Verification items for the finished model (mm, model axes). A direction names the side the tool comes from. Round coordinates to 2 decimals unless told otherwise and drop trailing zeros. Loops run counter-clockwise (first coordinate to the right, second up) from the corner with the lowest first, then second, coordinate; pieces in that order, holes last. Notation, with made-up numbers: M 71.5,-19 L 113.5,-19 A27 ccw 113.5,9 Z; hole C 19,58 d3. An arc over 180 degrees is marked long. Write item = value, one per line. Start each with the question number.
from build123d import *

# Parameters (mm, degrees)
ESQUISSE1_W             = 30
ESQUISSE1_H             = 30
BOSS_EXTRU_1_DEPTH      = 30
ESQUISSE2_W             = 20
ESQUISSE2_H             = 20
ENL_V_MAT_EXTRU_1_DEPTH = 31
ESQUISSE3_W             = 20
ESQUISSE3_H             = 20
ENL_V_MAT_EXTRU_2_DEPTH = 31
ESQUISSE4_W             = 20
ESQUISSE4_H             = 20
ENL_V_MAT_EXTRU_3_DEPTH = 31


with BuildPart() as part:
    # Esquisse1 → Boss.-Extru.1 (new body)
    with BuildSketch(Plane.XY):
        with Locations((15, 15)):
            Rectangle(ESQUISSE1_W, ESQUISSE1_H)
    extrude(amount=BOSS_EXTRU_1_DEPTH)

    # Esquisse2 → Enlèv. mat.-Extru.1 (cut, through all)
    with BuildSketch(Plane(origin=(0, 30, 0), x_dir=(1, 0, 0), z_dir=(0, 1, 0))):
        with Locations((15, -15)):
            Rectangle(ESQUISSE2_W, ESQUISSE2_H)
    extrude(amount=-ENL_V_MAT_EXTRU_1_DEPTH, mode=Mode.SUBTRACT)

    # Esquisse3 → Enlèv. mat.-Extru.2 (cut, through all)
    with BuildSketch(Plane.XY.offset(30)):
        with Locations((15, 15)):
            Rectangle(ESQUISSE3_W, ESQUISSE3_H)
    extrude(amount=-ENL_V_MAT_EXTRU_2_DEPTH, mode=Mode.SUBTRACT)

    # Esquisse4 → Enlèv. mat.-Extru.3 (cut, through all)
    with BuildSketch(Plane(origin=(30, 0, 0), x_dir=(0, 0, -1), z_dir=(1, 0, 0))):
        with Locations((-15, 15)):
            Rectangle(ESQUISSE4_W, ESQUISSE4_H)
    extrude(amount=-ENL_V_MAT_EXTRU_3_DEPTH, mode=Mode.SUBTRACT)


solid = part.part
1. Tool access check on faces 1 (the flat face through (3, 15, 25)), 2 (the flat face through (25, 15, 3)), 3 (the flat face through (25, 3, 15)). Record the directions out of +Z, -Z, +X, -X, +Y, -Y that give a thin tool (end or side, any length) a straight path to the whole face; none if there is none.
2. Section check C-C, the plane x = 27.5. Enter the section's corners in (y, z), and give its area (3 significant figures).
3. Gauge pin test, flat end, axial feed: P1, Ø4, axis at x = 8, z = 16, coming from the -Y side. Record the tip position at first contact, or that the pin passes through.
4. Section check A-A, the plane z = 8.5. Enter the section's corners in (x, y).
5. Mould release check, pull along Z, two halves, no side actions. Record for faces 4 (the flat face through (4.8, 15.2, 30)), 5 (the flat face through (15, 5, 28)), 6 (the flat face through (5, 28, 15)), 7 (the flat face through (3, 5, 15)): pulls with the +Z half, pulls with the -Z half, needs draft (parallel to the pull), parting line crosses it, or undercut.
6. Thickness scan on line 1 (Z direction, x = 27.5, y = 10). Record the ranges inside material, lowest first.
Computed values:
q1.face_1 = +X, -X
q1.face_2 = +Z, -Z
q1.face_3 = +Y, -Y
q2.outline = M 0,0 L 30,0 L 30,30 L 0,30 Z; hole M 5,5 L 25,5 L 25,25 L 5,25 Z
q2.area = 500 mm2
q3.P1 = through
q4.outline = M 0,0 L 5,0 L 5,5 L 0,5 Z; M 0,25 L 5,25 L 5,30 L 0,30 Z; M 25,0 L 30,0 L 30,5 L 25,5 Z; M 25,25 L 30,25 L 30,30 L 25,30 Z
q5.face_4 = pulls with the +Z half
q5.face_5 = needs draft
q5.face_6 = undercut
q5.face_7 = undercut
q6.line_1 = 0 to 5, 25 to 30
